Verification items for this drawing (mm, ordinates from the low corner). Give positions to 0.01 mm unless a question says otherwise; leave off trailing zeros. Loops run counter-clockwise (first coordinate to the right, second up) from the corner with the lowest first, then second, coordinate; pieces in that order, holes last. Notation, with made-up numbers: M 83.5,-23.5 L 109.5,-23.5 A27 ccw 109.5,10.5 Z; hole C 22,75 d2. An arc over 180 degrees is marked long. Answer in a Markdown table with one row per item.
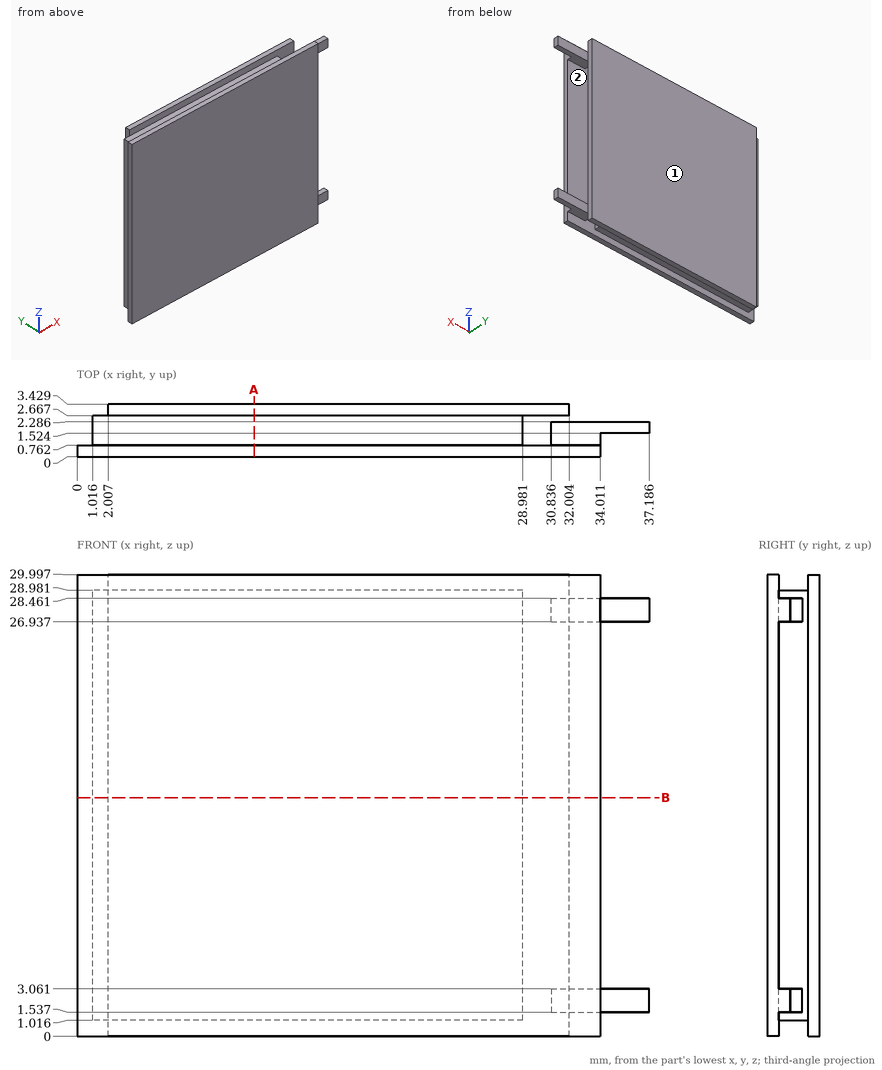
Item 1: Scan lines: L1, parallel to X at y = 1.25, z = 27.5 (1 decimal); L2, parallel to Y at x = 31, z = 21.5; L3, parallel to Z at x = 11, y = 0.95. Record each from-to range of solid material in increasing order. Write a range as [from, to].
Reported:
| item | result |
|---|---|
| L1 | x = [1, 29], [30.8, 34] |
| L2 | y = [0, 0.76], [2.67, 3.43] |
| L3 | z = [1.02, 28.98] |
Item 2: Sectioned sample at B-B (z = 15.5). Record the cut outline in (x, y), and give its area (3 significant figures).
Reported:
| item | result |
|---|---|
| outline | M 0,0 L 34.01,0 L 34.01,0.76 L 28.98,0.76 L 28.98,2.67 L 32,2.67 L 32,3.43 L 2.01,3.43 L 2.01,2.67 L 1.02,2.67 L 1.02,0.76 L 0,0.76 Z |
| area | 102 mm^2 |
Item 3: Sectioned sample at A-A (x = 11.5). Record the cut outline in (y, z).
Reported:
| item | result |
|---|---|
| outline | M 0,0 L 0.76,0 L 0.76,1.02 L 2.67,1.02 L 2.67,0 L 3.43,0 L 3.43,30 L 2.67,30 L 2.67,28.98 L 0.76,28.98 L 0.76,30 L 0,30 Z |
Item 4: Go/stop test with flat-tipped pins: pin 1 (0.6 mm diameter, centred on y = 1.5, z = 10.5, fed in from +X); pin 2 (0.5 mm diameter, centred on y = 1.5, z = 2, fed in from -X); pin 3 (1.2 mm diameter, centred on x = 34, z = 2.5, fed in from +Y). Record where each tip stops, or that it passes through.
Reported:
| item | result |
|---|---|
| pin 1 | stops at x = 28.98 |
| pin 2 | stops at x = 1.02 |
| pin 3 | stops at y = 2.29 |
Item 5: Release check for a two-part mould opening along Z. For the marked faces 1 and 2 record: released by +Z, released by -Z, zero draft, split by the parting line, or undercut.
Reported:
| item | result |
|---|---|
| face 1 | zero draft |
| face 2 | undercut |
